from build123d import *

# Parameters (mm, degrees)
BOSS_EXTRUDE1_DEPTH = 10
SKETCH2_R           = 4
BOSS_EXTRUDE2_DEPTH = 10
LPATTERN1_COUNT     = 2
LPATTERN1_PITCH     = 40
LPATTERN2_COUNT     = 2
LPATTERN2_PITCH     = 140
LPATTERN4_COUNT     = 2
LPATTERN4_PITCH     = 160


with BuildPart() as part:
    # Sketch1 → Boss-Extrude1 (new body)
    with BuildSketch(Plane(origin=(0, 0, 0), x_dir=(1, 0, 0), z_dir=(0, 1, 0))):
        Polygon((-125, 90.549169605), (125, 90.549169605), (125, 60.549169605), (-10, 60.549169605), (-10, -109.450830395), (125, -109.450830395), (125, -139.450830395), (-125, -139.450830395), (-125, -109.450830395), (-60, -109.450830395), (-60, 60.549169605), (-125, 60.549169605), align=None)
    extrude(amount=BOSS_EXTRUDE1_DEPTH)

    # Sketch2 → Boss-Extrude2 (add)
    with BuildSketch(Plane.ZY.offset(60)):
        with BuildLine():
            Line((115.450830395, 10), (133.450830395, 10))
            Line((133.450830395, 10), (133.450830395, 35))
            ThreePointArc((133.450830395, 35), (124.450830395, 44), (115.450830395, 35))
            Line((115.450830395, 35), (115.450830395, 10))
        make_face()
        with Locations((124.450830395, 35)):
            Circle(SKETCH2_R, mode=Mode.SUBTRACT)
    boss_extrude2 = extrude(amount=-BOSS_EXTRUDE2_DEPTH)

    # LPattern1: Boss-Extrude2 ×2
    with Locations(*[(i * LPATTERN1_PITCH, 0, 0) for i in range(1, LPATTERN1_COUNT)]):
        add(boss_extrude2)

    # LPattern2: Boss-Extrude2 ×2
    with Locations(*[(i * LPATTERN2_PITCH, 0, 0) for i in range(1, LPATTERN2_COUNT)]):
        add(boss_extrude2)

    # LPattern4: Boss-Extrude2 ×2
    with Locations(*[(i * LPATTERN4_PITCH, 0, 0) for i in range(1, LPATTERN4_COUNT)]):
        add(boss_extrude2)


solid = part.part
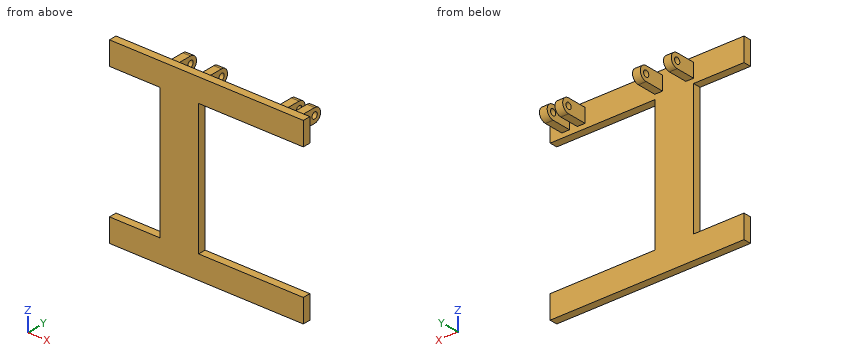
Check sheet for the modelled part. Datum: model origin and axes. Units: mm. Give positions to 0.01 mm unless a question says otherwise; leave off trailing zeros. Write each loop counter-clockwise with the first axis right and the second up, starting at its lowest first coordinate (ties: lowest second). Pieces come first, ordered by that corner, then holes. Notation, with made-up numbers: (-35, -23.5) -> (-29, -23.5) arc R27 ccw to (-29, 4.5) -> close; hole circle Ø9 at (-6.5, 61). An arc over 180 degrees is marked (long way). One line per item, written item: value. Start each with the question number.
Item 1: Section check B-B on y = 16. Record the cut outline in (x, z).
Item 2: Gauge pin test, flat ends, axial feed: pin 1 (9 mm diameter, centred on y = 31.5, z = 123, fed in from +X); pin 2 (11 mm diameter, centred on x = -56, y = 25, fed in from +Z); pin 3 (5 mm diameter, centred on x = 106.5, y = 22, fed in from -Z). Record the tip position at first contact, or that the pin passes through.
Item 3: Material ranges on probe 1 along Y at (x, z) = (-41.5, 124); probe 2 along Z at (x, y) = (81.5, 13), recorded low to high. Write a range as from..to.
Item 4: Section check D-D on z = 50. Record the cut outline in (x, y), then the cut area to 3 significant figures.
Item 5: Section check A-A on x = 36.5. Record the cut outline in (y, z), then the cut area to 3 significant figures.
Item 6: Section check C-C on x = -15. Record the cut outline in (y, z).
Results list:
1. outline: (-60, 115.45) -> (-50, 115.45) -> (-50, 133.45) -> (-60, 133.45) -> close; (-20, 115.45) -> (-10, 115.45) -> (-10, 133.45) -> (-20, 133.45) -> close; (80, 115.45) -> (90, 115.45) -> (90, 133.45) -> (80, 133.45) -> close; (100, 115.45) -> (110, 115.45) -> (110, 133.45) -> (100, 133.45) -> close
2. pin 1: x = 110
2. pin 2: z = 133.45
2. pin 3: z = 115.45
3. probe 1: 0..10
3. probe 2: 115.45..133.45
4. outline: (-60, 0) -> (-10, 0) -> (-10, 10) -> (-60, 10) -> close
4. area: 500 mm²
5. outline: (0, -90.55) -> (10, -90.55) -> (10, -60.55) -> (0, -60.55) -> close; (0, 109.45) -> (10, 109.45) -> (10, 139.45) -> (0, 139.45) -> close
5. area: 600 mm²
6. outline: (0, -90.55) -> (10, -90.55) -> (10, 115.45) -> (35, 115.45) arc R9 ccw to (35, 133.45) -> (10, 133.45) -> (10, 139.45) -> (0, 139.45) -> close; hole circle Ø8 at (35, 124.45)
